```python
from build123d import *

# Parameters (mm, degrees)
F_3_48_TAPPED_HOLE1_D = 1.9939
CIRPATTERN1_COUNT     = 12
BOSS_EXTRUDE1_DEPTH   = 3.175


with BuildPart() as part:
    # Cross Section → Main (revolve)
    with BuildSketch(Plane.XY):
        with BuildLine():
            Line((-38.1, 0), (-38.1, -3.175))
            Line((-38.1, -3.175), (-39.6367, -3.175))
            Line((-39.6367, -3.175), (-39.6367, -15.875))
            Line((-39.6367, -15.875), (-42.8117, -15.875))
            Line((-42.8117, -15.875), (-42.8117, -3.175))
            Line((-42.8117, -3.175), (-49.6697, -3.175))
            Line((-49.6697, -3.175), (-49.6697, 9.525))
            Line((-49.6697, 9.525), (-48.26, 9.525))
            Line((-48.26, 9.525), (-48.26, 1.5875))
            Line((-48.26, 1.5875), (-39.6875, 1.5875))
            ThreePointArc((-39.6875, 1.5875), (-38.564967985, 1.122532015), (-38.1, 0))
        make_face()
    revolve(axis=Axis((0, 55, 0), (0, -1, 0)))

    # #3-48 Tapped Hole1 (through all)
    with Locations(Plane(origin=(0, 1.5875, 0), x_dir=(1, 0, 0), z_dir=(0, 1, 0))):
        with Locations((-43.97375, 0)):
            f_3_48_tapped_hole1 = Hole(F_3_48_TAPPED_HOLE1_D / 2)

    # CirPattern1: #3-48 Tapped Hole1 ×12 about axis
    cirpattern1_axis = Axis((0, 0, 0), (0, 1, 0))
    for i in range(1, CIRPATTERN1_COUNT):
        add(f_3_48_tapped_hole1.rotate(cirpattern1_axis, i * 360 / CIRPATTERN1_COUNT), mode=Mode.SUBTRACT)

    # Sketch3 → Boss-Extrude1 (add)
    with BuildSketch(Plane(origin=(0, 1.5875, 0), x_dir=(1, 0, 0), z_dir=(0, 1, 0))):
        with BuildLine():
            Line((-45.692838455, -15.530361037), (-41.202710394, -11.040232976))
            Line((-41.202710394, -11.040232976), (-47.336339391, -9.39673204))
            ThreePointArc((-47.336339391, -9.39673204), (-46.615580377, -12.490607117), (-45.692838455, -15.530361037))
        make_face()
    extrude(amount=BOSS_EXTRUDE1_DEPTH)


solid = part.part
```
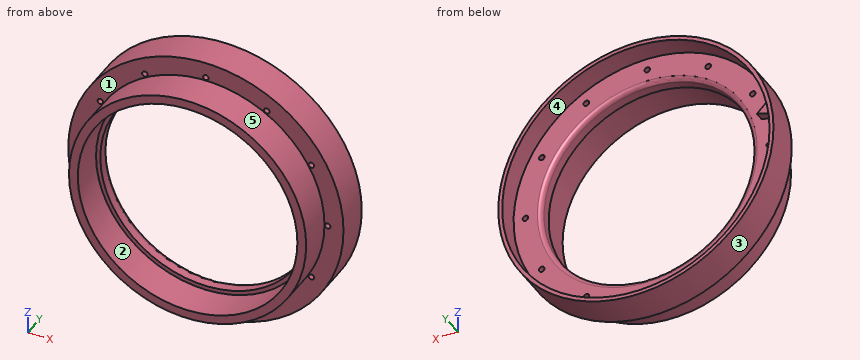
Input: part model. Units: mm. Frame: model coordinates. Face numbers are marked on the shaded views. A direction names the side the tool comes from. Give positions to 0.01 mm unless a question says otherwise; leave off trailing zeros. Order: outer loops, then holes, each group sorted by start corner. A loop starts at its lowest first (then second) coordinate and runs counter-clockwise, first axis right, second up. Notation, with made-up numbers: (54, 10) - (113, 10) arc R29 cw to (113, 39) - close; hole circle Ø7 at (69, 49.25). An arc over 180 degrees is marked (long way). One line per item, written item: value.
1. Reachability of the marked faces 4 and 5 from +Z, -Z, +X, -X, +Y, -Y: full face, straight path, thin tool, end or side. Return the list, or none.
Determined:
face 4: +Y
face 5: -Y
2. Cut plane A-A, the plane y = -11. Output: boundary loops of the cut face in (x, z).
Determined:
outline: circle Ø85.62 at (0, 0); hole circle Ø79.27 at (0, 0)
3. Draft query along X for the marked faces 1, 2 and 3. Return one class per face: released by +X, released by -X, zero draft, split by the parting line, or undercut.
Determined:
face 1: zero draft
face 2: undercut
face 3: split by the parting line
4. Pin query (flat end, axial travel): pin 1 Ø8 at (y, z) = (-12.5, -37) entering from -X; pin 2 Ø3 at (x, z) = (38.08, 21.99) entering from +Y; pin 3 Ø5 at (x, y) = (-2, 4.5) entering from -Z; pin 4 Ø1.2 at (x, z) = (21.99, -38.08) entering from -Y. Return the tip coordinate at first contact, or that it passes through.
Determined:
pin 1: x = -27.27
pin 2: y = 1.59
pin 3: z = -49.67
pin 4: through
5. Line query: probe 1 along X at (y, z) = (6.75, 0); probe 2 along Z at (x, y) = (0, -11.25); probe 3 along Z at (x, y) = (-3, -2). Output: solid intervals per line, ascending.
Determined:
probe 1: -49.67 to -48.26, 48.26 to 49.67
probe 2: -42.81 to -39.64, 39.64 to 42.81
probe 3: -49.58 to -37.98, 37.98 to 49.58
